```python
from build123d import *

# Parameters (mm, degrees)
EXTRUDE_1_DEPTH          = 7.5
CUT_EXTRUDE_1_DEPTH      = 27.249846584
CUT_EXTRUDE_1_DEPTH_BACK = 27.249846584
SKETCH_2_R               = 4.2
CUT_EXTRUDE_2_DEPTH      = 27.516200545
CUT_EXTRUDE_2_DEPTH_BACK = 27.516200545
SKETCH_3_R               = 4.2
FILLET_1_R               = 7.5
SKETCH_4_R               = 4.2
SKETCH_4_R_2             = 3.5
EXTRUDE_2_DEPTH          = 0.8
SKETCH_5_R               = 4.2
SKETCH_5_R_2             = 3.5
EXTRUDE_3_DEPTH          = 0.8


with BuildPart() as part:
    # ｽｹｯﾁ1 → ﾎﾞｽ - 押し出し1 (new, symmetric)
    with BuildSketch(Plane.XY):
        Polygon((0, 0), (-14.150635095, 8.169872981), (-11.650635095, 12.5), (1.339745962, 5), (6.339745962, 5), (19.330127019, 12.5), (21.830127019, 8.169872981), (7.679491924, 0), align=None)
    extrude(amount=EXTRUDE_1_DEPTH, both=True)

    # ｽｹｯﾁ2 → ｶｯﾄ - 押し出し1 (cut, two sides: drawn at the far end of the back side and taken through both)
    with BuildSketch(Plane(origin=(0, 0, 0), x_dir=(0, 0, 1), z_dir=(-0.5000000000000012, -0.866025403784438, 0)).offset(-CUT_EXTRUDE_1_DEPTH_BACK)):
        with Locations(Location((0, 8.839745962, 0), (0, 0, 270))):
            Circle(SKETCH_2_R)
    extrude(amount=CUT_EXTRUDE_1_DEPTH + CUT_EXTRUDE_1_DEPTH_BACK, mode=Mode.SUBTRACT)

    # ｽｹｯﾁ3 → ｶｯﾄ - 押し出し2 (cut, two sides: drawn at the far end of the back side and taken through both)
    with BuildSketch(Plane(origin=(1.919872981, -3.325317547, 0), x_dir=(0, 0, -1), z_dir=(0.5000000000000013, -0.8660254037844379, 0)).offset(-CUT_EXTRUDE_2_DEPTH_BACK)):
        with Locations(Location((0, 15.490381057, 0), (0, 0, 90))):
            Circle(SKETCH_3_R)
    extrude(amount=CUT_EXTRUDE_2_DEPTH + CUT_EXTRUDE_2_DEPTH_BACK, mode=Mode.SUBTRACT)

    # ﾌｨﾚｯﾄ1
    fillet_1_edges = [part.edges().sort_by_distance(p)[0] for p in [
        (20.580127019, 10.334936491, -7.5),
        (20.580127019, 10.334936491, 7.5),
        (-12.900635095, 10.334936491, -7.5),
        (-12.900635095, 10.334936491, 7.5),
    ]]
    fillet(fillet_1_edges, radius=FILLET_1_R - 0.0001)  # a hair under: the kernel refuses the full size

    # ｽｹｯﾁ4 → ﾎﾞｽ - 押し出し2 (add)
    with BuildSketch(Plane(origin=(0, 0, 0), x_dir=(0.8660254037844382, -0.500000000000001, 0), z_dir=(0.5000000000000009, 0.866025403784438, 0))):
        with Locations((-8.839745962, 0)):
            Circle(SKETCH_4_R)
        with Locations((-8.839745962, 0)):
            Circle(SKETCH_4_R_2, mode=Mode.SUBTRACT)
    extrude(amount=EXTRUDE_2_DEPTH)

    # ｽｹｯﾁ5 → ﾎﾞｽ - 押し出し3 (add)
    with BuildSketch(Plane(origin=(1.919872981, -3.325317547, 0), x_dir=(0.8660254037844378, 0.5000000000000017, 0), z_dir=(-0.5000000000000016, 0.8660254037844377, 0))):
        with Locations((15.490381057, 0)):
            Circle(SKETCH_5_R)
        with Locations((15.490381057, 0)):
            Circle(SKETCH_5_R_2, mode=Mode.SUBTRACT)
    extrude(amount=EXTRUDE_3_DEPTH)


solid = part.part
```
CAD build for the part. Positions are in the model's coordinates, mm. A direction names the side the tool comes from. Coordinates: 2 decimals unless noted, no trailing zeros. Order: outer loops, then holes, each group sorted by start corner. A loop starts at its lowest first (then second) coordinate and runs counter-clockwise, first axis right, second up. Notation, with made-up numbers: (-33, -4) - (21, -4) arc R30 cw to (21, 19) - close; hole circle Ø11 at (12.5, -25.5). An arc over 180 degrees is marked (long way). Use a Markdown table: item, result. Add a question column.
(1) Saw through at C-C (z = -4.75). Give the cut face in (x, y).
(2) Flat gauge pins, fed straight in: pin 1 (4 mm diameter, centred on x = 3.5, z = 1, fed in from +Y); pin 2 (1 mm diameter, centred on x = 16, z = 2, fed in from +Y); pin 3 (1 mm diameter, centred on x = 9, y = 8.5, fed in from -Z); pin 4 (4 mm diameter, centred on y = 4, z = 3.5, fed in from +X). Where does each tip first touch, or does it go through?
(3) Saw through at D-D (y = 1.5). Give the cut face in (x, z).
(4) Saw through at A-A (z = -2.5). Give the cut face in (x, y), then the cut area to 3 significant figures.
(5) Drill centre lines: line 1 along X through (y, z) = (7.5, 3.75); line 2 along Y through (x, z) = (6, -3.25); line 3 along X through (y, z) = (6, -2). Where is each one in solid material? Low to high. Write a range as [from, to].
(6) Pull direction Y, two halves, no side cores. Call faces 3 (the face through (-2.36, 7.136, -3.228)), 4 (the face through (-2.721, 4.954, 1.262)), 5 (the face through (17.23, 8.9, -1.61)), 6 (the face through (4, 0, 0)): +Y half, -Y half, draft (parallel to the pull), parting line (faces both ways), or undercut.
(7) Saw through at B-B (z = 1.5). Give the cut face in (x, y).
(8) Which spindle directions (+Z, -Z, +X, -X, +Y, -Y) get a long thin tool onto all of the face, cutting with end or side? Do faces 1 (the face through (-4.57, 3.09, -1.05)), 2 (the face through (9.857, 7.031, -3.228)). Say none if no direction does.
Solved:
| question | item | result |
|---|---|---|
| 1 | outline | (-12.68, 7.32) - (0, 0) - (7.68, 0) - (20.36, 7.32) - (17.86, 11.65) - (6.34, 5) - (1.34, 5) - (-10.18, 11.65) - close |
| 2 | pin 1 | stops at y = 5 |
| 2 | pin 2 | stops at y = 10.87 |
| 2 | pin 3 | passes through |
| 2 | pin 4 | stops at x = 18.07 |
| 3 | outline | (-2.6, -7.5) - (10.28, -7.5) - (10.28, 7.5) - (-2.6, 7.5) - close |
| 4 | outline | (-13.78, 7.96) - (-9.78, 5.64) - (-9.38, 6.34) - (-10.18, 6.8) - (-8.08, 10.44) - (-11.28, 12.29) - close; (-5.53, 3.2) - (0, 0) - (7.68, 0) - (13.21, 3.2) - (12.81, 3.89) - (12.01, 3.43) - (9.91, 7.06) - (6.34, 5) - (1.34, 5) - (-2.23, 7.06) - (-4.33, 3.43) - (-5.13, 3.89) - close; (15.76, 10.44) - (17.86, 6.8) - (17.06, 6.34) - (17.46, 5.64) - (21.46, 7.96) - (18.96, 12.29) - close |
| 4 | area | 120 mm² |
| 5 | line 1 | x = [-12.99, -8.06], [-3.69, -2.99], [10.67, 11.37], [15.74, 20.67] |
| 5 | line 2 | y = [0, 5] |
| 5 | line 3 | x = [-10.39, -10.06], [-2.48, -0.39], [8.07, 10.16], [17.74, 18.07] |
| 6 | face 3 | +Y half |
| 6 | face 4 | undercut |
| 6 | face 5 | undercut |
| 6 | face 6 | -Y half |
| 7 | outline | (-14.02, 8.09) - (-10.39, 6) - (-9.99, 6.69) - (-10.65, 7.07) - (-8.55, 10.71) - (-11.52, 12.42) - close; (-4.92, 2.84) - (0, 0) - (7.68, 0) - (12.6, 2.84) - (12.2, 3.53) - (11.54, 3.15) - (9.44, 6.79) - (6.34, 5) - (1.34, 5) - (-1.76, 6.79) - (-3.86, 3.15) - (-4.52, 3.53) - close; (16.23, 10.71) - (18.33, 7.07) - (17.67, 6.69) - (18.07, 6) - (21.7, 8.09) - (19.2, 12.42) - close |
| 8 | face 1 | none |
| 8 | face 2 | +Z, -Z, +Y |
